Check sheet for the modelled part. Datum: model origin and axes. Units: mm. A direction names the side the tool comes from. Give positions to 0.01 mm unless a question says otherwise; leave off trailing zeros. Write each loop counter-clockwise with the first axis right and the second up, starting at its lowest first coordinate (ties: lowest second). Pieces come first, ordered by that corner, then holes. Notation, with made-up numbers: (49, -7.75) -> (96, -7.75) arc R20 cw to (96, 8.25) -> close; hole circle Ø10 at (46, 55.25). An arc over 180 degrees is marked (long way). Use a Markdown table: item, result. Add a question column.
1. Release check for a two-part mould opening along Y. For faces 1 (the cylindrical face through (23.846, 7.509, 35.185)), 2 (the flat face through (0, 0, 13)), 3 (the flat face through (11, -11, 58)) record: released by +Y, released by -Y, zero draft, split by the parting line, or undercut.
2. Gauge pin test, flat ends, axial feed: P1, Ø3, axis at x = -10, y = 41.5, coming from the +Z side; P2, Ø1.5, axis at x = -8, z = 44.5, coming from the +Y side; P3, Ø11.5, axis at x = 22.5, y = 38.97, coming from the -Z side; P4, Ø2, axis at x = 0, z = 42, coming from the -Y side. Record the tip position at first contact, or that the pin passes through.
3. Cross-section at C-C (x = 0). Enter the section's corners in (y, z).
4. Scan lines: probe 1 along Y at (x, z) = (0, 32.5); probe 2 along Y at (x, z) = (22.5, 7); probe 3 along Z at (x, y) = (37, 26.5). Record each from-to range of solid material in increasing order. Write a range as [from, to].
5. Set-up check for faces 4 (the cylindrical face through (21.85, 43.93, 6.41)), 5 (the flat face through (28, 1, 13)): record each of +Z, -Z, +X, -X, +Y, -Y from which the full face is reachable in a straight line by a thin tool's end or side.
6. Cross-section at A-A (y = 0). Enter the section's corners in (x, z), then the cut area to 3 significant figures.
7. Cross-section at D-D (z = 29.5). Enter the section's corners in (x, y), then the cut area to 3 significant figures.
8. Cross-section at B-B (x = 22.5). Enter the section's corners in (y, z).
from build123d import *

# Parameters (mm, degrees)
SKETCH_R      = 65
SKETCH_R_2    = 5
PAD_DEPTH     = 13
SKETCH001_R   = 25
SKETCH001_R_2 = 15
PAD001_DEPTH  = 45


with BuildPart() as part:
    # Sketch → Pad (new body)
    with BuildSketch(Plane.XY):
        Circle(SKETCH_R)
        with Locations((22.5, 38.971143)):
            Circle(SKETCH_R_2, mode=Mode.SUBTRACT)
        with Locations((-45, 0)):
            Circle(SKETCH_R_2, mode=Mode.SUBTRACT)
        with Locations((22.5, -38.971143)):
            Circle(SKETCH_R_2, mode=Mode.SUBTRACT)
    extrude(amount=PAD_DEPTH)

    # Sketch001 (on Face6 of Pad) → Pad001 (join)
    with BuildSketch(Plane.XY.offset(13)):
        Circle(SKETCH001_R)
        Circle(SKETCH001_R_2, mode=Mode.SUBTRACT)
    extrude(amount=PAD001_DEPTH)


solid = part.part
Worked answers:
| question | item | result |
|---|---|---|
| 1 | face 1 | split by the parting line |
| 1 | face 2 | undercut |
| 1 | face 3 | zero draft |
| 2 | P1 | stops at z = 13 |
| 2 | P2 | stops at y = 23.93 |
| 2 | P3 | stops at z = 0 |
| 2 | P4 | stops at y = -25 |
| 3 | outline | (-65, 0) -> (65, 0) -> (65, 13) -> (25, 13) -> (25, 58) -> (15, 58) -> (15, 13) -> (-15, 13) -> (-15, 58) -> (-25, 58) -> (-25, 13) -> (-65, 13) -> close |
| 4 | probe 1 | y = [-25, -15], [15, 25] |
| 4 | probe 2 | y = [-60.98, -43.97], [-33.97, 33.97], [43.97, 60.98] |
| 4 | probe 3 | z = [0, 13] |
| 5 | face 4 | +Z, -Z |
| 5 | face 5 | +Z |
| 6 | outline | (-65, 0) -> (-50, 0) -> (-50, 13) -> (-65, 13) -> close; (-40, 0) -> (65, 0) -> (65, 13) -> (25, 13) -> (25, 58) -> (15, 58) -> (15, 13) -> (-15, 13) -> (-15, 58) -> (-25, 58) -> (-25, 13) -> (-40, 13) -> close |
| 6 | area | 2,460 mm² |
| 7 | outline | circle Ø50 at (0, 0); hole circle Ø30 at (0, 0) |
| 7 | area | 1,260 mm² |
| 8 | outline | (-60.98, 0) -> (-43.97, 0) -> (-43.97, 13) -> (-60.98, 13) -> close; (-33.97, 0) -> (33.97, 0) -> (33.97, 13) -> (10.9, 13) -> (10.9, 58) -> (-10.9, 58) -> (-10.9, 13) -> (-33.97, 13) -> close; (43.97, 0) -> (60.98, 0) -> (60.98, 13) -> (43.97, 13) -> close |
